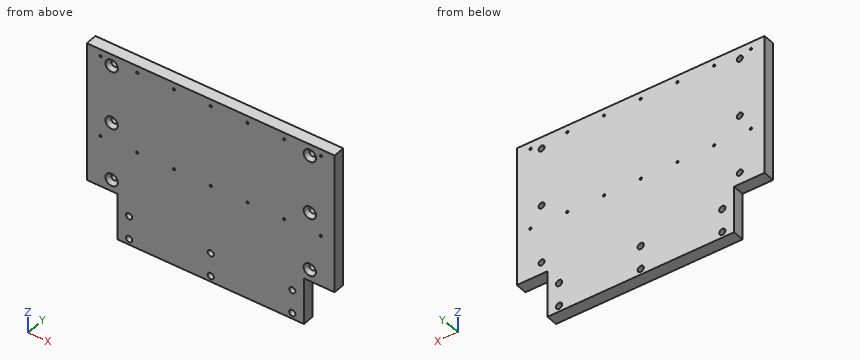
```python
from build123d import *

# Parameters (mm, degrees)
F0_W           = 269.875
F0_H           = 203.2
F1_DEPTH       = 12.7
F2_W           = 33.3375
F2_H           = 50.8
F3_DEPTH       = 12.7
F5_D           = 6.7564
F7_D           = 2.5
F7_DEPTH       = 20.55
F7_TIP         = 0.7510757738
F9_D           = 6.5278
F9_CSINK_D     = 13.4874
F9_CSINK_ANGLE = 82


# Not quite as in the source:
# - a feature names something its author has since deleted; it is built from what else it names


with BuildPart() as f1:
    # F0 (on Front) → F1 (new body)
    with BuildSketch(Plane.XZ):
        with Locations((134.9375, 101.6)):
            Rectangle(F0_W, F0_H)
    extrude(amount=F1_DEPTH)

    # F2 (on face) → F3 (cut, through all)
    with BuildSketch(Plane.XZ.offset(12.7)):
        with Locations((16.66875, 25.4)):
            Rectangle(F2_W, F2_H)
        with Locations((253.20625, 25.4)):
            Rectangle(F2_W, F2_H)
    extrude(amount=-F3_DEPTH, mode=Mode.SUBTRACT)

    # F5 (through all)
    with Locations(Plane.XZ.offset(12.7)):
        with Locations((223.8375, 31.75), (223.8375, 6.35), (134.9375, 6.35), (134.9375, 31.75), (46.0375, 31.75), (46.0375, 6.35)):
            Hole(F5_D / 2)

    # F7
    with Locations(Plane.XZ.offset(12.7)):
        with Locations((54.9375, 195.7), (94.9375, 195.7), (134.9375, 195.7), (174.9375, 195.7), (214.9375, 195.7), (214.9375, 106.8), (174.9375, 106.8), (134.9375, 106.8), (94.9375, 106.8), (54.9375, 106.8), (14.9375, 195.7), (14.9375, 106.8), (254.9375, 195.7), (254.9375, 106.8)):
            Hole(F7_D / 2, depth=F7_DEPTH)
            with Locations((0, 0, -(F7_DEPTH + F7_TIP / 2))):  # 118° drill point
                Cone(0, F7_D / 2, F7_TIP, mode=Mode.SUBTRACT)

    # F9 (through all)
    with Locations(Plane.XZ.offset(12.7)):
        with Locations((26.9875, 190.5), (26.9875, 127), (26.9875, 63.5), (242.8875, 63.5), (242.8875, 127), (242.8875, 190.5)):
            CounterSinkHole(F9_D / 2, F9_CSINK_D / 2, counter_sink_angle=F9_CSINK_ANGLE)


solid = f1.part
```
Geometry check sheet. Reference: the model listing, model coordinates, mm. Give positions to 0.01 mm unless a question says otherwise; leave off trailing zeros. Order: outer loops, then holes, each group sorted by start corner. A loop starts at its lowest first (then second) coordinate and runs counter-clockwise, first axis right, second up.
1. Section check A-A, the plane z = 6.35. Enter the section's corners in (x, y).
2. Section check B-B, the plane z = 63.5. Enter the section's corners in (x, y) (3 decimals), and give its area (3 significant figures).
3. Gauge pin test, flat ends, axial feed: pin 1 Ø1.5 at (x, z) = (214.94, 106.8) entering from +Y; pin 2 Ø7.5 at (x, z) = (26.99, 127) entering from -Y; pin 3 Ø1.5 at (y, z) = (-4, 45.5) entering from +X; pin 4 Ø1.5 at (y, z) = (-7, 40.5) entering from -X. Record the tip position at first contact, or that the pin passes through.
4. Section check C-C, the plane y = -5.5. Give the number of separate pieces and of enclosed holes in the cut face, and give its area (3 significant figures).
5. Thickness scan on L1, parallel to X at y = -4.25, z = 63.5 (3 decimals); L2, parallel to Z at x = 134, y = -10.5; L3, parallel to Z at x = 14, y = -12. Record the ranges inside material, lowest first.
Values follow:
1. outline: (33.34, -12.7) - (42.66, -12.7) - (42.66, 0) - (33.34, 0) - close; (49.42, -12.7) - (131.56, -12.7) - (131.56, 0) - (49.42, 0) - close; (138.32, -12.7) - (220.46, -12.7) - (220.46, 0) - (138.32, 0) - close; (227.22, -12.7) - (236.54, -12.7) - (236.54, 0) - (227.22, 0) - close
2. outline: (0, -12.7) - (20.244, -12.7) - (23.724, -8.697) - (23.724, 0) - (0, 0) - close; (30.251, -8.697) - (33.731, -12.7) - (236.144, -12.7) - (239.624, -8.697) - (239.624, 0) - (30.251, 0) - close; (246.151, -8.697) - (249.631, -12.7) - (269.875, -12.7) - (269.875, 0) - (246.151, 0) - close
2. area: 3,230 mm2
3. pin 1: passes through
3. pin 2: stops at y = -9.26
3. pin 3: stops at x = 236.54
3. pin 4: stops at x = 33.34
4. separate pieces: 1
4. enclosed holes: 26
4. area: 51,000 mm2
5. L1: x = 0 to 23.724, 30.251 to 239.624, 246.151 to 269.875
5. L2: z = 0 to 3.1, 9.6 to 28.5, 35 to 105.97, 107.63 to 194.87, 196.53 to 203.2
5. L3: z = 50.8 to 105.97, 107.63 to 194.87, 196.53 to 203.2
